Design review of the part built by this model. Coordinates are the model's own, in mm. Face numbers are marked on the shaded views. Round coordinates to 2 decimals unless told otherwise and drop trailing zeros. Loops run counter-clockwise (first coordinate to the right, second up) from the corner with the lowest first, then second, coordinate; pieces in that order, holes last. Notation, with made-up numbers: (76.5, 74) - (94.5, 74) arc R15 ccw to (94.5, 96) - close; hole circle Ø2 at (-20.5, -3.75). An arc over 180 degrees is marked (long way). Answer as CSV lines item,"result". Start each with the question number.
(1) Consider section B-B (z = 150.5). Give the boundary of the cut face in (x, y) (1 decimal), and give its area (3 significant figures).
(2) Consider section C-C (x = -13.5). Give the boundary of the cut face in (y, z), and give its area (3 significant figures).
(3) For P1, Ø12, axis at x = -35.5, z = 441.5, coming from the -Y side; P2, Ø5, axis at y = -5.5, z = 318.5, coming from the +X side; P3, Ø6, axis at x = 38.5, z = 308, coming from the -Y side, all flat-tipped, find the tip position at first contact; note any pin that passes through.
(4) Mouldability with a two-part tool opening along Y and no side actions: class the marked faces 1 and 2 as released by +Y, released by -Y, zero draft, split by the parting line, or undercut.
(5) Consider section A-A (y = 0). Give the boundary of the cut face in (x, z).
(6) Wall thickness on L1, parallel to Y at x = 0, z = 259; L2, parallel to X at y = -41.5, z = 395; L3, parallel to X at y = -31, z = 483.5: over which ranges is each line inside the solid? List them lowest first.
(7) Consider section D-D (z = 554). Give the boundary of the cut face in (x, y) (1 decimal), and give its area (3 significant figures).
from build123d import *

# Parameters (mm, degrees)
SKETCH1_R           = 50.8
SKETCH1_R_2         = 49.2125
BOSS_EXTRUDE1_DEPTH = 660.4
CUT_EXTRUDE3_START  = 51.1937
SKETCH4_W           = 2.9972
SKETCH4_H           = 25.4
CUT_EXTRUDE3_DEPTH  = 151.6126


with BuildPart() as part:
    # Sketch1 → Boss-Extrude1 (new body)
    with BuildSketch(Plane.XY):
        Circle(SKETCH1_R)
        Circle(SKETCH1_R_2, mode=Mode.SUBTRACT)
    extrude(amount=BOSS_EXTRUDE1_DEPTH)

    # Sketch4 → Cut-Extrude3 (cut)
    with BuildSketch(Plane.XY.offset(CUT_EXTRUDE3_START)):
        Polygon((54.24331314, -33.04782567), (32.246267884, -20.34782567), (33.744867884, -17.75217433), (55.74191314, -30.45217433), align=None)
        with Locations((0, 50.8)):
            Rectangle(SKETCH4_W, SKETCH4_H)
        Polygon((-55.74191314, -30.45217433), (-33.744867884, -17.75217433), (-32.246267884, -20.34782567), (-54.24331314, -33.04782567), align=None)
    extrude(amount=CUT_EXTRUDE3_DEPTH, mode=Mode.SUBTRACT)


solid = part.part
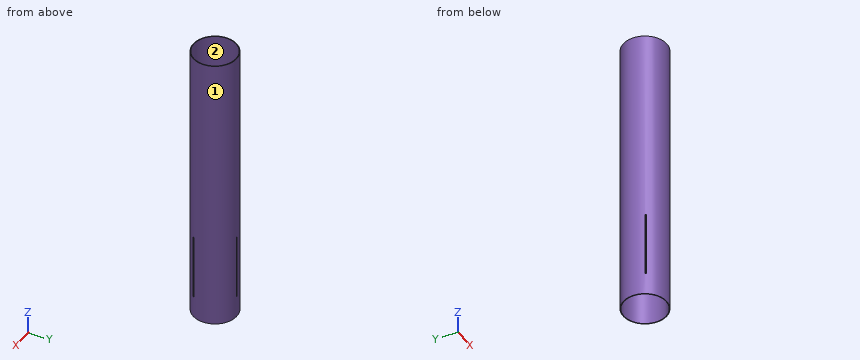
Determined:
1,outline,"(-44.7, -24.1) - (-43.3, -23.3) arc R49.2 cw to (-1.5, 49.2) - (-1.5, 50.8) arc R50.8 ccw to start; (-43.2, -26.7) arc R50.8 ccw to (43.2, -26.7) - (41.9, -25.9) arc R49.2 cw to (-41.9, -25.9) - close; (1.5, 49.2) arc R49.2 cw to (43.3, -23.3) - (44.7, -24.1) arc R50.8 ccw to (1.5, 50.8) - close"
1,area,"485 mm^2"
2,outline,"(-48.97, 0) - (-47.32, 0) - (-47.32, 660.4) - (-48.97, 660.4) - close; (47.32, 0) - (48.97, 0) - (48.97, 660.4) - (47.32, 660.4) - close"
2,area,"2,180 mm^2"
3,P1,"stops at y = -41.36"
3,P2,"stops at x = 50.71"
3,P3,"stops at y = -36.34"
4,face 1,"split by the parting line"
4,face 2,"undercut"
5,outline,"(-50.8, 0) - (-49.21, 0) - (-49.21, 660.4) - (-50.8, 660.4) - close; (49.21, 0) - (50.8, 0) - (50.8, 660.4) - (49.21, 660.4) - close"
6,L1,"y = -50.8 to -49.21, 49.21 to 50.8"
6,L2,"x = -29.3 to -26.45, 26.45 to 29.3"
6,L3,"x = -40.24 to -38.22, 38.22 to 40.24"
7,outline,"circle Ø101.6 at (0, 0); hole circle Ø98.4 at (0, 0)"
7,area,"499 mm^2"
